Can you work these out from the model? Positions are in its coordinate system, mm. Face numbers are marked on the shaded views. A direction names the side the tool comes from. Round coordinates to 2 decimals unless told otherwise and drop trailing zeros. Write each loop counter-clockwise with the first axis right and the second up, starting at its lowest first coordinate (ties: lowest second). Pieces come first, ordered by that corner, then holes. Notation, with made-up numbers: M 31,70 L 41,70 A19 ccw 41,100 Z; hole C 7.5,65.25 d7. An arc over 180 degrees is marked long. Answer in a Markdown table with one row per item. Add a question column.
(1) I'm going to push flat-ended pins straight in: pin 1 (0.6 mm diameter, centred on y = -2, z = -1, fed in from +X) (3 decimals); pin 2 (4 mm diameter, centred on x = 8, z = 2, fed in from -Y); pin 3 (0.8 mm diameter, centred on y = -2.5, z = 1.5, fed in from -X) (3 decimals); pin 4 (0.8 mm diameter, centred on x = -7.5, z = 1.5, fed in from +Y). Where does each tip first touch, or does it pass through?
(2) Suppose I cut it at B-B, the plane y = 8.25. Write out the boundary of the cut face in (x, z), then the cut area to 3 significant figures.
(3) Suppose I cut it at C-C, the plane x = -7.5. Write out the boundary of the cut face in (y, z) (3 decimals).
(4) For the marked faces 4 and 5, which set-ups out of +Z, -Z, +X, -X, +Y, -Y let a thin tool reach every point of the face, with its end or its side?
(5) Suppose I cut it at D-D, the plane y = 6.25. Count the separate pieces of the cut face and the enclosed holes in it, then the cut area to 3 significant figures.
(6) If I drill on probe 1 along X at (y, z) = (7.75, 3.75); probe 2 along Z at (x, y) = (7.5, -2.25) (3 decimals); probe 3 along Z at (x, y) = (5.75, 6), over which ranges is the centre line in solid material (lowest first)?
(7) If we mould it in two halves opening along Z, with no side actions, what happens to the marked faces 1, 2 and 3? For each: released by +Z, released by -Z, zero draft, split by the parting line, or undercut.
(8) Suppose I cut it at A-A, the plane z = -2.5. Write out the boundary of the cut face in (x, y).
from build123d import *

# Parameters (mm, degrees)
SKETCH_1_W           = 25.26
SKETCH_1_H           = 9
EXTRUDE_1_DEPTH      = 9
SKETCH_2_W           = 22.86
SKETCH_2_H           = 6.6
CUT_EXTRUDE_1_DEPTH  = 6.5
SKETCH_3_W           = 4.2
SKETCH_3_H           = 6.5
CUT_EXTRUDE_2_DEPTH  = 6.5
EXTRUDE_2_DEPTH      = 3.5
EXTRUDE_2_DEPTH_BACK = 8
SKETCH_5_W           = 0.75
SKETCH_5_H           = 0.75


with BuildPart() as part:
    # 草图1 → 拉伸1 (new body)
    with BuildSketch(Plane(origin=(0, 0, 0), x_dir=(1, 0, 0), z_dir=(0, 1, 0))):
        Rectangle(SKETCH_1_W, SKETCH_1_H)
    extrude(amount=EXTRUDE_1_DEPTH)

    # 草图2 → 切除-拉伸1 (cut)
    with BuildSketch(Plane(origin=(0, 9, 0), x_dir=(-1, 0, 0), z_dir=(0, 1, 0))):
        Rectangle(SKETCH_2_W, SKETCH_2_H)
    extrude(amount=-CUT_EXTRUDE_1_DEPTH, mode=Mode.SUBTRACT)

    # 草图3 → 切除-拉伸2 (cut)
    with BuildSketch(Plane.XY.offset(4.5)):
        with Locations((0, 5.75)):
            Rectangle(SKETCH_3_W, SKETCH_3_H)
    extrude(amount=-CUT_EXTRUDE_2_DEPTH, mode=Mode.SUBTRACT)

    # 草图5 → 拉伸2 (add, two sides: drawn at the far end of the back side and taken through both)
    with BuildSketch(Plane.XZ.offset(-EXTRUDE_2_DEPTH_BACK)):
        with Locations((0, 1.27)):
            Rectangle(SKETCH_5_W, SKETCH_5_H)
        with Locations((2.54, 1.27)):
            Rectangle(SKETCH_5_W, SKETCH_5_H)
        with Locations((5.08, 1.27)):
            Rectangle(SKETCH_5_W, SKETCH_5_H)
        with Locations((7.62, 1.27)):
            Rectangle(SKETCH_5_W, SKETCH_5_H)
        with Locations((-2.54, 1.27)):
            Rectangle(SKETCH_5_W, SKETCH_5_H)
        with Locations((-5.08, 1.27)):
            Rectangle(SKETCH_5_W, SKETCH_5_H)
        with Locations((-7.62, 1.27)):
            Rectangle(SKETCH_5_W, SKETCH_5_H)
        with Locations((-7.62, -1.27)):
            Rectangle(SKETCH_5_W, SKETCH_5_H)
        with Locations((-5.08, -1.27)):
            Rectangle(SKETCH_5_W, SKETCH_5_H)
        with Locations((-2.54, -1.27)):
            Rectangle(SKETCH_5_W, SKETCH_5_H)
        with Locations((7.62, -1.27)):
            Rectangle(SKETCH_5_W, SKETCH_5_H)
        with Locations((5.08, -1.27)):
            Rectangle(SKETCH_5_W, SKETCH_5_H)
        with Locations((2.54, -1.27)):
            Rectangle(SKETCH_5_W, SKETCH_5_H)
        with Locations((0, -1.27)):
            Rectangle(SKETCH_5_W, SKETCH_5_H)
    extrude(amount=EXTRUDE_2_DEPTH + EXTRUDE_2_DEPTH_BACK)


solid = part.part
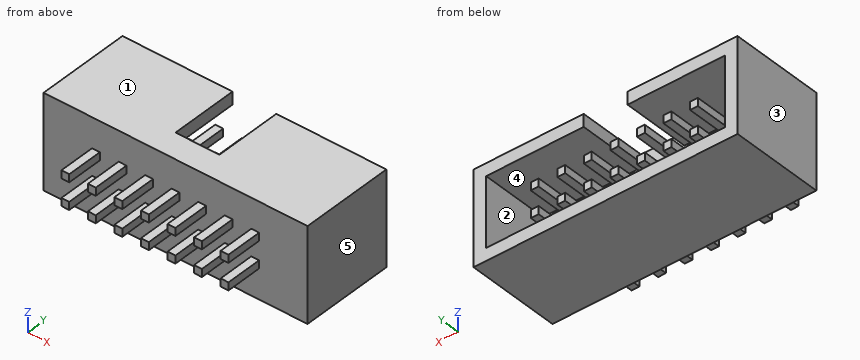
Calculated:
| question | item | result |
|---|---|---|
| 1 | pin 1 | x = 7.995 |
| 1 | pin 2 | y = -3.5 |
| 1 | pin 3 | x = -7.995 |
| 1 | pin 4 | y = 8 |
| 2 | outline | M -12.63,-4.5 L 12.63,-4.5 L 12.63,4.5 L 2.1,4.5 L 2.1,3.3 L 11.43,3.3 L 11.43,-3.3 L -11.43,-3.3 L -11.43,3.3 L -2.1,3.3 L -2.1,4.5 L -12.63,4.5 Z |
| 2 | area | 71.4 mm² |
| 3 | outline | M -3.5,-1.645 L 0,-1.645 L 0,-4.5 L 9,-4.5 L 9,-3.3 L 2.5,-3.3 L 2.5,-1.645 L 8,-1.645 L 8,-0.895 L 2.5,-0.895 L 2.5,0.895 L 8,0.895 L 8,1.645 L 2.5,1.645 L 2.5,3.3 L 9,3.3 L 9,4.5 L 0,4.5 L 0,1.645 L -3.5,1.645 L -3.5,0.895 L 0,0.895 L 0,-0.895 L -3.5,-0.895 Z |
| 4 | face 4 | +Y |
| 4 | face 5 | +Z, -Z, +X, +Y, -Y |
| 5 | separate pieces | 15 |
| 5 | enclosed holes | 0 |
| 5 | area | 79.3 mm² |
| 6 | probe 1 | -12.63 to -2.1, 2.1 to 12.63 |
| 6 | probe 2 | -1.645 to -0.895, 0.895 to 1.645 |
| 6 | probe 3 | -4.5 to -3.3, 3.3 to 4.5 |
| 7 | face 1 | released by +Z |
| 7 | face 2 | undercut |
| 7 | face 3 | zero draft |
| 8 | outline | M -12.63,0 L 12.63,0 L 12.63,9 L 11.43,9 L 11.43,2.5 L -11.43,2.5 L -11.43,9 L -12.63,9 Z |
